Source: CAD feature listing. Evaluate the final solid. Frame: model axes, mm. Face numbers are marked on the shaded views. Round coordinates to 2 decimals unless told otherwise and drop trailing zeros. Write each loop counter-clockwise with the first axis right and the second up, starting at its lowest first coordinate (ties: lowest second). Pieces come first, ordered by that corner, then holes.
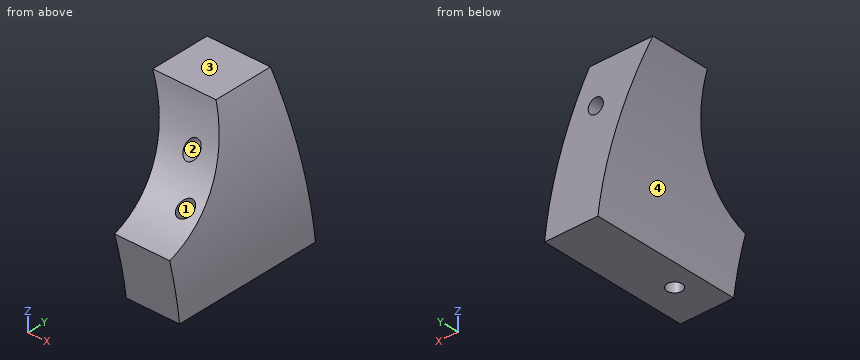
```python
from build123d import *

# Parameters (mm, degrees)
BOSS_EXTRUDE1_DEPTH      = 60
SKETCH25_W               = 5.5
SKETCH25_H               = 17
BOSS_EXTRUDE3_DEPTH      = 20
FILLET1_R                = 2.3
SKETCH28_W               = 8
SKETCH28_H               = 10
CUT_EXTRUDE17_DEPTH      = 265
CUT_EXTRUDE19_DEPTH      = 165.638713704
CUT_EXTRUDE19_DEPTH_BACK = 165.638713704
SKETCH30_W               = 183.61
SKETCH30_H               = 30
CUT_EXTRUDE20_DEPTH      = 165.638713704
CUT_EXTRUDE20_DEPTH_BACK = 165.638713704
SKETCH32_W               = 3
SKETCH32_H               = 14
BOSS_EXTRUDE4_DEPTH      = 40
CUT_EXTRUDE21_DEPTH      = 164.320868385
CUT_EXTRUDE21_DEPTH_BACK = 164.320868385
CUT_EXTRUDE22_DEPTH      = 164.320868502
CUT_EXTRUDE22_DEPTH_BACK = 164.320868502
SKETCH40_W               = 31.800896411
SKETCH40_H               = 59.801829262
CUT_EXTRUDE23_DEPTH      = 55
SKETCH41_R               = 2
CUT_EXTRUDE24_DEPTH      = 55
SKETCH42_R               = 2
CUT_EXTRUDE25_DEPTH      = 55


with BuildPart() as part:
    # Sketch1 → Boss-Extrude1 (new body)
    with BuildSketch(Plane(origin=(0, 0, 0), x_dir=(1, 0, 0), z_dir=(0, 1, 0))):
        with BuildLine():
            Line((91.805, -10), (90.252689849, -10))
            ThreePointArc((90.252689849, -10), (0, -90.805), (-90.252689849, -10))
            Line((-90.252689849, -10), (-91.805, -10))
            Line((-91.805, -10), (-91.805, 20))
            Line((-91.805, 20), (-76.805, 20))
            Line((-76.805, 20), (-76.805, 0))
            ThreePointArc((-76.805, 0), (0, -76.805), (76.805, 0))
            Line((76.805, 0), (76.805, 20))
            Line((76.805, 20), (91.805, 20))
            Line((91.805, 20), (91.805, -10))
        make_face()
    extrude(amount=-BOSS_EXTRUDE1_DEPTH)

    # Sketch25 → Boss-Extrude3 (add)
    with BuildSketch(Plane(origin=(0, -60, 0), x_dir=(-1, 0, 0), z_dir=(0, -1, 0))):
        with Locations((84.305, 5)):
            Rectangle(SKETCH25_W, SKETCH25_H)
        with Locations((-84.305, 5)):
            Rectangle(SKETCH25_W, SKETCH25_H)
    extrude(amount=BOSS_EXTRUDE3_DEPTH)

    # Fillet1
    fillet1_edges = [part.edges().sort_by_distance(p)[0] for p in [
        (84.305, -60, 3.5),
        (81.555, -60, -5),
        (87.055, -60, -5),
        (84.305, -60, -13.5),
        (-84.305, -60, 3.5),
        (-87.055, -60, -5),
        (-81.555, -60, -5),
        (-84.305, -60, -13.5),
    ]]
    fillet(fillet1_edges, radius=FILLET1_R)

    # Sketch28 → Cut-Extrude17 (cut)
    with BuildSketch(Plane(origin=(91.805, 0, 0), x_dir=(0, 0, -1), z_dir=(1, 0, 0))):
        with Locations((5, -42)):
            Rectangle(SKETCH28_W, SKETCH28_H)
    extrude(amount=-CUT_EXTRUDE17_DEPTH, mode=Mode.SUBTRACT)

    # Sketch30 → Cut-Extrude19 (cut, two sides: drawn at the far end of the back side and taken through both)
    with BuildSketch(Plane(origin=(0, 0, -20), x_dir=(-1, 0, 0), z_dir=(0, 0, -1)).offset(-CUT_EXTRUDE19_DEPTH_BACK)):
        with Locations((0, -15)):
            Rectangle(SKETCH30_W, SKETCH30_H)
    extrude(amount=CUT_EXTRUDE19_DEPTH + CUT_EXTRUDE19_DEPTH_BACK, mode=Mode.SUBTRACT)

    # Sketch32 → Cut-Extrude20 (cut, two sides: drawn at the far end of the back side and taken through both)
    with BuildSketch(Plane(origin=(0, 0, -20), x_dir=(-1, 0, 0), z_dir=(0, 0, -1)).offset(-CUT_EXTRUDE20_DEPTH_BACK)):
        with Locations((-65.13523483, -44)):
            Rectangle(SKETCH32_W, SKETCH32_H)
        with Locations((-51.773928511, -44)):
            Rectangle(SKETCH32_W, SKETCH32_H)
        with Locations((-84.305, -46)):
            Rectangle(SKETCH32_W, SKETCH32_H)
        with Locations((65.13523483, -44)):
            Rectangle(SKETCH32_W, SKETCH32_H)
        with Locations((51.773928511, -44)):
            Rectangle(SKETCH32_W, SKETCH32_H)
        with Locations((84.305, -46)):
            Rectangle(SKETCH32_W, SKETCH32_H)
    extrude(amount=CUT_EXTRUDE20_DEPTH + CUT_EXTRUDE20_DEPTH_BACK, mode=Mode.SUBTRACT)

    # Sketch33 → Boss-Extrude4 (add)
    with BuildSketch(Plane(origin=(0, -60, 0), x_dir=(-1, 0, 0), z_dir=(0, -1, 0))):
        with BuildLine():
            ThreePointArc((-90.252689849, -10), (-84.815671791, -32.432234638), (-73.898492454, -52.768938193))
            Line((-73.898492454, -52.768938193), (-61.590580503, -45.886909008))
            ThreePointArc((-61.590580503, -45.886909008), (-71.169996018, -28.876282513), (-76.151218145, -10))
            Line((-76.151218145, -10), (-90.252689849, -10))
        make_face()
        with BuildLine():
            ThreePointArc((73.898492454, -52.768938193), (84.815671791, -32.432234638), (90.252689849, -10))
            Line((90.252689849, -10), (76.151218145, -10))
            ThreePointArc((76.151218145, -10), (71.169996018, -28.876282513), (61.590580503, -45.886909008))
            Line((61.590580503, -45.886909008), (73.898492454, -52.768938193))
        make_face()
    extrude(amount=BOSS_EXTRUDE4_DEPTH)

    # Sketch37 → Cut-Extrude21 (cut, two sides: drawn at the far end of the back side and taken through both)
    with BuildSketch(Plane(origin=(0, 0, 0), x_dir=(0, 0, -1), z_dir=(1, 0, 0)).offset(-CUT_EXTRUDE21_DEPTH_BACK)):
        with BuildLine():
            Line((-0.881303102, -100), (-23.690614963, -100))
            ThreePointArc((-23.690614963, -100), (-31.684760451, -85.14357588), (-45.886909008, -76.037606625))
            Line((-45.886909008, -76.037606625), (-45.886909008, -59.917167305))
            Line((-45.886909008, -59.917167305), (-66.948234535, -59.917167305))
            Line((-66.948234535, -59.917167305), (-63.746381293, -92.441906362))
            Line((-63.746381293, -92.441906362), (-47.571757556, -115.346464391))
            Line((-47.571757556, -115.346464391), (-8.086377987, -115.346464391))
            Line((-8.086377987, -115.346464391), (-0.881303102, -100))
        make_face()
    extrude(amount=CUT_EXTRUDE21_DEPTH + CUT_EXTRUDE21_DEPTH_BACK, mode=Mode.SUBTRACT)

    # Sketch38 → Cut-Extrude22 (cut, two sides: drawn at the far end of the back side and taken through both)
    with BuildSketch(Plane(origin=(0, 0, 0), x_dir=(0, 0, -1), z_dir=(1, 0, 0)).offset(-CUT_EXTRUDE22_DEPTH_BACK)):
        Polygon((20, -30), (-90.805, -30), (-90.805, -60), (-10, -60), (-10, -100), (20, -100), (20, -60), align=None)
    extrude(amount=CUT_EXTRUDE22_DEPTH + CUT_EXTRUDE22_DEPTH_BACK, mode=Mode.SUBTRACT)


with BuildPart() as cut_extrude22_piece_1:
    # of the separate pieces the step leaves, piece 1, a body of its own (cut_extrude22_pieces)
    add(part.part.solids().sort_by_distance((76.151218145, -60, 10))[0])

    # Sketch41 → Cut-Extrude24 (cut)
    with BuildSketch(Plane(origin=(0, 0, 10), x_dir=(-1, 0, 0), z_dir=(0, 0, -1))):
        with Locations((-82.252689849, -89.36002802)):
            Circle(SKETCH41_R)
    extrude(amount=-CUT_EXTRUDE24_DEPTH, mode=Mode.SUBTRACT)

    # Sketch42 → Cut-Extrude25 (cut)
    with BuildSketch(Plane(origin=(0, -60, 0), x_dir=(1, 0, 0), z_dir=(0, 1, 0))):
        with Locations(Location((76.708608453, -36.023832562, 0), (0, 0, 270))):
            Circle(SKETCH42_R)
    extrude(amount=-CUT_EXTRUDE25_DEPTH, mode=Mode.SUBTRACT)


with BuildPart() as cut_extrude22_piece_2:
    # of the separate pieces the step leaves, piece 2, a body of its own (cut_extrude22_pieces)
    add(part.part.solids().sort_by_distance((-76.151218145, -60, 10))[0])

    # Sketch40 → Cut-Extrude23 (cut)
    with BuildSketch(Plane(origin=(0, -100, 0), x_dir=(-1, 0, 0), z_dir=(0, -1, 0))):
        with Locations((74.352241644, -39.900914631)):
            Rectangle(SKETCH40_W, SKETCH40_H)
    extrude(amount=-CUT_EXTRUDE23_DEPTH, mode=Mode.SUBTRACT)


solid = cut_extrude22_piece_1.part
```
Q1. Section query A-A, the plane z = 37. Output: boundary loops of the cut face in (x, y).
Q2. Line query: line 1 (Y direction, x = 81, z = 26); line 2 (Z direction, x = 77.25, y = -61.5); line 3 (Z direction, x = 78.75, y = -67). Output: solid intervals per line, ascending.
Q3. Mould query, pull axis X, two halves, no side actions, for the marked faces 1, 2, 3 and 4. Classes: pulls with the +X half, pulls with the -X half, needs draft (parallel to the pull), parting line crosses it, or undercut.
Q4. Pin query (flat end, axial travel): P1, Ø4, axis at x = 68.5, y = -66.5, coming from the -Z side; P2, Ø8, axis at y = -90, z = 31, coming from the -X side; P3, Ø5, axis at x = 67.5, z = 35.5, coming from the -Y side; P4, Ø6.5, axis at x = 76.71, z = 36.02, coming from the +Y side. Return the tip coordinate at first contact, or that it passes through.
Q5. Section query B-B, the plane y = -65.5. Output: boundary loops of the cut face in (x, z) (3 decimals), and give its area (3 significant figures).
Q6. Section query C-C, the plane z = 22. Output: boundary loops of the cut face in (x, y).
Q7. Section query D-D, the plane x = 64.75. Output: boundary loops of the cut face in (y, z), and give its area (3 significant figures).
Filled in:
1. outline: (67.31, -80.5) - (74.96, -80.5) - (74.96, -60) - (67.31, -60) - close; (78.45, -80.5) - (82.92, -80.5) - (82.92, -60) - (78.45, -60) - close
2. line 1: y = -93.52 to -90.92, -87.8 to -60
2. line 2: z = 10 to 34.1, 37.95 to 45.89
2. line 3: z = 10 to 45.21
3. face 1: undercut
3. face 2: undercut
3. face 3: needs draft
3. face 4: pulls with the -X half
4. P1: stops at z = 30.48
4. P2: stops at x = 70.31
4. P3: stops at y = -83.27
4. P4: stops at y = -60
5. outline: (61.591, 45.887) arc R76.805 cw to (76.151, 10) - (90.253, 10) arc R90.805 ccw to (78.358, 45.887) - close; hole circle Ø4 at (76.709, 36.024)
5. area: 527 mm2
6. outline: (73.59, -100) - (88.1, -100) - (88.1, -60) - (73.59, -60) - close; hole circle Ø4 at (82.25, -89.36)
7. outline: (-77.92, 41.31) - (-60, 41.31) - (-60, 45.89) - (-76.04, 45.89) arc R33.63 cw to start
7. area: 77.4 mm2
